```python
from build123d import *

# Parameters (mm, degrees)
SKETCH1_R           = 8.5
BOSS_EXTRUDE1_DEPTH = 3
BOSS_EXTRUDE2_DEPTH = 3
CIRPATTERN2_COUNT   = 12
FILLET5_R           = 6
FILLET6_R           = 6
BOSS_EXTRUDE3_DEPTH = 3
FILLET9_R           = 2.5
SKETCH20_R          = 3.6
CUT_EXTRUDE11_DEPTH = 10
SKETCH21_R          = 0.5
CUT_EXTRUDE12_DEPTH = 10
BOSS_EXTRUDE4_DEPTH = 3
SKETCH23_R          = 1.25
CUT_EXTRUDE13_DEPTH = 3
FILLET10_R          = 5
FILLET11_R          = 2


# Some blends are built 0.0001 mm under size
with BuildPart() as part:
    # Sketch1 → Boss-Extrude1 (new body)
    with BuildSketch(Plane.XY):
        Circle(SKETCH1_R)
    extrude(amount=BOSS_EXTRUDE1_DEPTH)

    # Sketch3 → Boss-Extrude2 (add)
    with BuildSketch(Plane.XY.offset(3)):
        Polygon((-1.305261922, 9.914448614), (-1.509060022, 7), (1.509060022, 7), (1.305261922, 9.914448614), (0.678518537, 11), (-0.678518537, 11), align=None)
    boss_extrude2 = extrude(amount=-BOSS_EXTRUDE2_DEPTH)

    # CirPattern2: Boss-Extrude2 ×12 about axis
    cirpattern2_axis = Axis((0, 0, 0), (0, 0, 1))
    for i in range(1, CIRPATTERN2_COUNT):
        add(boss_extrude2.rotate(cirpattern2_axis, i * 360 / CIRPATTERN2_COUNT))

    # Fillet5
    # the kernel refuses this fillet: 6 mm, written as the material it takes off along each edge
    with BuildSketch(Plane(origin=(9.238795325, 3.826834324, 6.454382408), x_dir=(0.4999999999998129, 0.8660254037845467, 0), z_dir=(0, 0, -1)), Plane(origin=(1.305261922, 9.914448614, 6.454382408), x_dir=(-0.5000000000001841, 0.8660254037843323, 0), z_dir=(0, 0, -1)), Plane(origin=(-7.933533403, 6.08761429, 6.454382408), x_dir=(-1, 0, 0), z_dir=(0, 0, -1)), Plane(origin=(-9.914448614, 1.305261922, 6.454382408), x_dir=(-0.8660254037843317, -0.5000000000001852, 0), z_dir=(0, 0, -1)), Plane(origin=(-9.238795325, -3.826834324, 6.454382408), x_dir=(-0.49999999999981826, -0.8660254037845436, 0), z_dir=(0, 0, -1)), Plane(origin=(-6.08761429, -7.933533403, 6.454382408), x_dir=(0, -1, 0), z_dir=(0, 0, -1)), Plane(origin=(3.826834324, -9.238795325, 6.454382408), x_dir=(0.866025403784545, -0.49999999999981576, 0), z_dir=(0, 0, -1)), Plane(origin=(7.933533403, -6.08761429, 6.454382408), x_dir=(1, 0, 0), z_dir=(0, 0, -1)), Plane(origin=(9.914448614, -1.305261922, 6.454382408), x_dir=(0.8660254037843321, 0.5000000000001844, 0), z_dir=(0, 0, -1))) as fillet5_piece_1:
        with BuildLine():
            CenterArc((1.388315544, -5.998484909), FILLET5_R, 91.287628333, 24.712371667)
            Line((-1.241911337, -0.605720631), (-1.294515874, -0.497865346))
            Line((-1.294515874, -0.497865346), (-0.052604538, 0.107855286))
            Line((-0.052604538, 0.107855286), (0, 0.12))
            ThreePointArc((0, 0.12), (0.626743385, 0.12), (1.250790195, 0.119969698))
            Line((1.250790195, 0.119969698), (1.25348677, 0))
        make_face()
    extrude(amount=9.908764816, mode=Mode.SUBTRACT)
    with BuildSketch(Plane(origin=(6.08761429, 7.933533403, 6.454382408), x_dir=(-0.4383711467890806, -0.8987940462991654, 0), z_dir=(0, 0, -1)), Plane(origin=(-3.826834324, 9.238795325, 6.454382408), x_dir=(0.5591929034707435, -0.8290375725550441, 0), z_dir=(0, 0, -1)), Plane(origin=(-1.305261922, -9.914448614, 6.454382408), x_dir=(-0.06975647374412178, 0.9975640502598244, 0), z_dir=(0, 0, -1))) as fillet5_piece_2:
        with BuildLine():
            CenterArc((1.381752963, 6), FILLET5_R, 245.287628333, 24.712371667)
            Line((-1.126626446, 0.549492433), (-1.176794034, 0.440482282))
            ThreePointArc((-1.176794034, 0.440482282), (-0.615917761, 0.166890931), (-0.052604538, -0.107855286))
            Line((-0.052604538, -0.107855286), (0, -0.12))
            Line((0, -0.12), (1.381752963, -0.12))
            Line((1.381752963, -0.12), (1.381752963, 0))
        make_face()
    extrude(amount=9.908764816, mode=Mode.SUBTRACT)

    # Fillet6
    # the kernel refuses this fillet: 6 mm, written as the material it takes off along each edge
    with BuildSketch(Plane(origin=(7.933533403, 6.08761429, 6.454382408), x_dir=(-0.8987940462991681, -0.4383711467890748, 0), z_dir=(0, 0, -1)), Plane(origin=(3.826834324, 9.238795325, 6.454382408), x_dir=(-0.5591929034707512, -0.8290375725550386, 0), z_dir=(0, 0, -1)), Plane(origin=(-1.305261922, 9.914448614, 6.454382408), x_dir=(-0.06975647374412959, -0.9975640502598239, 0), z_dir=(0, 0, -1)), Plane(origin=(-6.08761429, 7.933533403, 6.454382408), x_dir=(0.43837114678907496, -0.8987940462991681, 0), z_dir=(0, 0, -1)), Plane(origin=(-9.238795325, 3.826834324, 6.454382408), x_dir=(0.8290375725550394, -0.5591929034707502, 0), z_dir=(0, 0, -1)), Plane(origin=(-9.914448614, -1.305261922, 6.454382408), x_dir=(0.9975640502598241, -0.06975647374412908, 0), z_dir=(0, 0, -1)), Plane(origin=(-7.933533403, -6.08761429, 6.454382408), x_dir=(0.8987940462991686, 0.4383711467890744, 0), z_dir=(0, 0, -1)), Plane(origin=(-3.826834324, -9.238795325, 6.454382408), x_dir=(0.559192903470749, 0.8290375725550401, 0), z_dir=(0, 0, -1)), Plane(origin=(1.305261922, -9.914448614, 6.454382408), x_dir=(0.06975647374412973, 0.9975640502598241, 0), z_dir=(0, 0, -1)), Plane(origin=(6.08761429, -7.933533403, 6.454382408), x_dir=(-0.4383711467890742, 0.8987940462991686, 0), z_dir=(0, 0, -1)), Plane(origin=(9.238795325, -3.826834324, 6.454382408), x_dir=(-0.8290375725550386, 0.5591929034707512, 0), z_dir=(0, 0, -1)), Plane(origin=(9.914448614, 1.305261922, 6.454382408), x_dir=(-0.9975640502598239, 0.06975647374412945, 0), z_dir=(0, 0, -1))) as fillet6_piece_1:
        with BuildLine():
            CenterArc((1.381752963, -6), FILLET6_R, 90, 24.712371667)
            Line((-1.126626446, -0.549492433), (-1.176794034, -0.440482282))
            ThreePointArc((-1.176794034, -0.440482282), (-0.615917761, -0.166890931), (-0.052604538, 0.107855286))
            Line((-0.052604538, 0.107855286), (0, 0.12))
            Line((0, 0.12), (1.381752963, 0.12))
            Line((1.381752963, 0.12), (1.381752963, 0))
        make_face()
    extrude(amount=9.908764816, mode=Mode.SUBTRACT)

    # Sketch4 → Boss-Extrude3 (add)
    with BuildSketch(Plane(origin=(0, 0, 0), x_dir=(-1, 0, 0), z_dir=(0, 0, -1))):
        with BuildLine():
            Line((-2.5, 25.5), (-2.5, 4.330127019))
            ThreePointArc((-2.5, 4.330127019), (-5, 0), (-2.5, -4.330127019))
            Line((-2.5, -4.330127019), (-2.5, -7))
            Line((-2.5, -7), (2.5, -7))
            Line((2.5, -7), (2.5, -4.330127019))
            ThreePointArc((2.5, -4.330127019), (5, 0), (2.5, 4.330127019))
            Line((2.5, 4.330127019), (2.5, 25.5))
            Line((2.5, 25.5), (-2.5, 25.5))
        make_face()
    extrude(amount=-BOSS_EXTRUDE3_DEPTH)

    # Fillet9
    fillet9_edges = [part.edges().sort_by_distance(p)[0] for p in [
        (-2.5, 25.5, 1.5),
        (2.5, 25.5, 1.5),
    ]]
    fillet(fillet9_edges, radius=FILLET9_R - 0.0001)  # a hair under: the kernel refuses the full size

    # Sketch20 → Cut-Extrude11 (cut)
    with BuildSketch(Plane.XY.offset(3)):
        Circle(SKETCH20_R)
    extrude(amount=-CUT_EXTRUDE11_DEPTH, mode=Mode.SUBTRACT)

    # Sketch21 → Cut-Extrude12 (cut)
    with BuildSketch(Plane.XY.offset(3)):
        with Locations((0, 14.5)):
            Circle(SKETCH21_R)
        with Locations((0, 4.5)):
            Circle(SKETCH21_R)
        with Locations((0, 8.5)):
            Circle(SKETCH21_R)
    extrude(amount=-CUT_EXTRUDE12_DEPTH, mode=Mode.SUBTRACT)

    # Sketch22 → Boss-Extrude4 (add)
    with BuildSketch(Plane.XY.offset(3)):
        Polygon((0, 25.5), (6, 25.5), (6, 20.5), (-6, 20.5), (-6, 25.5), align=None)
    extrude(amount=-BOSS_EXTRUDE4_DEPTH)

    # Sketch23 → Cut-Extrude13 (cut)
    with BuildSketch(Plane.XY.offset(3)):
        with Locations((-3.5, 23)):
            Circle(SKETCH23_R)
        with Locations((3.5, 23)):
            Circle(SKETCH23_R)
    extrude(amount=-CUT_EXTRUDE13_DEPTH, mode=Mode.SUBTRACT)

    # Fillet10
    # the kernel refuses this fillet: 5 mm, written as the material it adds along each edge
    with BuildSketch(Plane(origin=(2.5, 20.5, 0), x_dir=(1, 0, 0), z_dir=(0, 0, 1))) as fillet10_piece_1:
        with BuildLine():
            CenterArc((5, -4.769696007), FILLET10_R, 107.457603124, 72.542396876)
            Line((0, -4.769696007), (-0.1, -4.769696007))
            Line((-0.1, -4.769696007), (-0.1, 0))
            Line((-0.1, 0), (0, 0.1))
            ThreePointArc((0, 0.1), (1.75, 0.1), (3.47, 0.09539392))
            Line((3.47, 0.09539392), (3.5, 0))
        make_face()
    extrude(amount=3)
    with BuildSketch(Plane(origin=(-2.5, 20.5, 3), x_dir=(0, -1, 0), z_dir=(0, 0, -1))) as fillet10_piece_2:
        with BuildLine():
            CenterArc((4.769696007, 5), FILLET10_R, 197.457603124, 72.542396876)
            Line((0, 3.5), (-0.09539392, 3.47))
            ThreePointArc((-0.09539392, 3.47), (-0.1, 1.75), (-0.1, 0))
            Line((-0.1, 0), (0, -0.1))
            Line((0, -0.1), (4.769696007, -0.1))
            Line((4.769696007, -0.1), (4.769696007, 0))
        make_face()
    extrude(amount=3)

    # Fillet11
    fillet11_edges = [part.edges().sort_by_distance(p)[0] for p in [
        (-6, 25.5, 1.5),
        (6, 25.5, 1.5),
    ]]
    fillet(fillet11_edges, radius=FILLET11_R)


solid = part.part
```
Source: CAD feature listing. Evaluate the final solid. Frame: model axes, mm. A direction names the side the tool comes from. Round coordinates to 2 decimals unless told otherwise and drop trailing zeros. Loops run counter-clockwise (first coordinate to the right, second up) from the corner with the lowest first, then second, coordinate; pieces in that order, holes last.
(1) Access query for faces 4 (the cylindrical face through (-7.889, -5.916, 1.521)), 5 (the cylindrical face through (-9.82, 1.17, 1.52)), 6 (the cylindrical face through (9.82, -1.17, 1.52)), 7 (the cylindrical face through (-7.924, 5.924, 1.521)), 8 (the cylindrical face through (-3.9, 9.09, 1.52)). Directions: +Z, -Z, +X, -X, +Y, -Y. A direction counts if a zero-diameter tool reaches every point of the face in a straight line with its end or side. Return the directions, or none.
From the geometry:
face 4: +Z, -Z, -Y
face 5: +Z, -Z, -X
face 6: +Z, -Z, +X
face 7: +Z, -Z, +Y
face 8: +Z, -Z
(2) Pull-direction query (Y, two-part tool) for faces 1 (the cylindrical face through (3.434, 1.081, 1.521)), 2 (the flat face through (6, 22, 2)), 3 (the cylindrical face through (7.889, 5.916, 1.521)); classes: +Y half, -Y half, draft (parallel to the pull), parting line (faces both ways), or undercut.
From the geometry:
face 1: undercut
face 2: draft
face 3: +Y half
(3) Contact query for flat-ended pins moving along their axis: pin 1 Ø0.9 at (y, z) = (13.5, 1.5) entering from -X; pin 2 Ø1 at (y, z) = (-3, 0.5) entering from -X; pin 3 Ø3 at (x, y) = (3.5, 23) entering from -Z; pin 4 Ø1.5 at (y, z) = (22.5, 1) entering from +X. Output: stop coordinate, or through.
From the geometry:
pin 1: stops at x = -2.5
pin 2: stops at x = -8.67
pin 3: stops at z = 0
pin 4: stops at x = 6
(4) Section query B-B (x = 0). Output: boundary loops of the cut face in (y, z).
From the geometry:
outline: (-11, 0) - (-3.6, 0) - (-3.6, 3) - (-11, 3) - close; (3.6, 0) - (4, 0) - (4, 3) - (3.6, 3) - close; (5, 0) - (8, 0) - (8, 3) - (5, 3) - close; (9, 0) - (14, 0) - (14, 3) - (9, 3) - close; (15, 0) - (25.5, 0) - (25.5, 3) - (15, 3) - close
(5) Section query A-A (y = 23). Output: boundary loops of the cut face in (x, z), and give its area (3 significant figures).
From the geometry:
outline: (-6, 0) - (-4.75, 0) - (-4.75, 3) - (-6, 3) - close; (-2.25, 0) - (2.25, 0) - (2.25, 3) - (-2.25, 3) - close; (4.75, 0) - (6, 0) - (6, 3) - (4.75, 3) - close
area: 21.0 mm2
(6) Material intervals for probe 1 along Y at (x, z) = (0, 0.6); probe 2 along X at (y, z) = (-9, 1.4); probe 3 along Y at (x, z) = (4.25, 0.3), sorted ascending.
From the geometry:
probe 1: y = -11 to -3.6, 3.6 to 4, 5 to 8, 9 to 14, 15 to 25.5
probe 2: x = -6.08 to -3.81, -1.35 to 1.35, 3.81 to 6.08
probe 3: y = -9.4 to 9.4, 19.53 to 22, 24 to 25.48
(7) Section query D-D (z = 0.65). Give the number of separate pieces and of enclosed holes in the cut face, and give its area (3 significant figures).
From the geometry:
separate pieces: 1
enclosed holes: 6
area: 366 mm2
(8) Section query C-C (y = 0). Output: boundary loops of the cut face in (x, z), and give its area (3 significant figures).
From the geometry:
outline: (-11, 0) - (-3.6, 0) - (-3.6, 3) - (-11, 3) - close; (3.6, 0) - (11, 0) - (11, 3) - (3.6, 3) - close
area: 44.4 mm2
